Can you work these out from the model? Positions are in its coordinate system, mm. Face numbers are marked on the shaded views. A direction names the side the tool comes from. Give positions to 0.01 mm unless a question says otherwise; leave off trailing zeros. Loops run counter-clockwise (first coordinate to the right, second up) from the corner with the lowest first, then second, coordinate; pieces in that order, holes last. Notation, with made-up numbers: (41.25, 84.5) - (96.25, 84.5) arc R6 cw to (96.25, 91.5) - close; hole circle Ø9 at (27, -2.5). An arc over 180 degrees is marked (long way). Answer as a JSON object with one key per item and string values. Group by question number.
Item 1: Which directions (+Z, -Z, +X, -X, +Y, -Y) give clear straight access to the entire face, cutting with the end or side of a thin tool? Please do the marked faces 1, 2 and 3.
Item 2: Suppose I cut it at D-D on x = -12. Write out the boundary of the cut face in (y, z).
Item 3: Suppose I cut it at A-A on y = 0. Write out the boundary of the cut face in (x, z).
Item 4: Will these pins go through, and if not, where does the flat tip stop? pin 1 (20 mm diameter, centred on x = 0, y = 0, fed in from +Z); pin 2 (3 mm diameter, centred on y = 16.5, z = 3, fed in from +X); pin 3 (3 mm diameter, centred on y = 5, z = 2, fed in from -X); pin 4 (2 mm diameter, centred on y = 12, z = 2.5, fed in from -X).
Item 5: Suppose I cut it at B-B on x = -25. Write out the boundary of the cut face in (y, z).
Item 6: Please list where these lines run through material, in increasing order: L1, parallel to X at y = 14.5, z = 6; L2, parallel to X at y = -16.5, z = 3; L3, parallel to Y at x = -3.5, z = 3.
Item 7: Thinking about a two-plate mould opening in X: for the marked faces 4, 5 and 6, which applies, pulls with the +X half, pulls with the -X half, needs draft (parallel to the pull), parting line crosses it, or undercut?
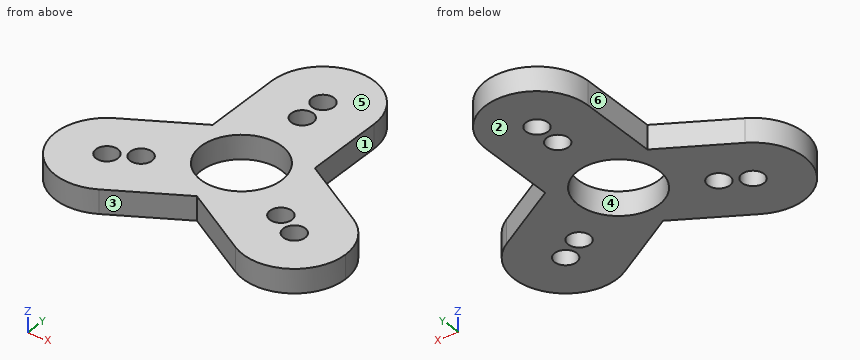
from build123d import *

# Parameters (mm, degrees)
F0_R     = 3
F0_R_2   = 11.05
F1_DEPTH = 6.5


with BuildPart() as f1:
    # F0 (on Top) → F1 (new body)
    with BuildSketch(Plane.XY):
        with BuildLine():
            ThreePointArc((-32.6519768305, -2.6858200754), (-37.7763321694, -21.8101758986), (-18.6519763031, -26.9345310768))
            ThreePointArc((-18.6519763031, -26.9345310768), (-13.5276209102, -21.8101754521), (-11.6519766687, -14.8101756349))
            ThreePointArc((-11.6519766687, -14.8101756349), (-18.6519767496, -2.6858199352), (-32.6519768305, -2.6858200754))
        make_face()
        with Locations((-25.6519766687, -14.8101756349)):
            Circle(F0_R, mode=Mode.SUBTRACT)
        with Locations((-19.1362317873, -11.0483085737)):
            Circle(F0_R, mode=Mode.SUBTRACT)
        with BuildLine():
            Line((0, -16.1658075373), (-7, -12.124355653))
            ThreePointArc((-7, -12.124355653), (-12.124355653, -7), (-14, 0))
            Line((-14, 0), (-14, 8.0829037687))
            Line((-14, 8.0829037687), (-32.6519768305, -2.6858200754))
            ThreePointArc((-32.6519768305, -2.6858200754), (-18.6519767496, -2.6858199352), (-11.6519766687, -14.8101756349))
            ThreePointArc((-11.6519766687, -14.8101756349), (-13.5276209102, -21.8101754521), (-18.6519763031, -26.9345310768))
            Line((-18.6519763031, -26.9345310768), (0, -16.1658075373))
        make_face()
        with BuildLine():
            Line((0, -16.1658075373), (7, -12.124355653))
            ThreePointArc((7, -12.124355653), (0, -14), (-7, -12.124355653))
            Line((-7, -12.124355653), (0, -16.1658075373))
        make_face()
        with BuildLine():
            ThreePointArc((39.6519766687, -14.8101756349), (37.7763323684, -7.8101757158), (32.6519768305, -2.6858200754))
            ThreePointArc((32.6519768305, -2.6858200754), (13.5276209927, -7.8101756747), (18.6519769101, -26.9345314273))
            ThreePointArc((18.6519769101, -26.9345314273), (32.6519767894, -26.9345312182), (39.6519766687, -14.8101756349))
        make_face()
        with Locations((19.1362317873, -11.0483085737)):
            Circle(F0_R, mode=Mode.SUBTRACT)
        with Locations((25.6519766687, -14.8101756349)):
            Circle(F0_R, mode=Mode.SUBTRACT)
        with BuildLine():
            Line((14, 8.0829037687), (14, 0))
            ThreePointArc((14, 0), (12.124355653, -7), (7, -12.124355653))
            Line((7, -12.124355653), (0, -16.1658075373))
            Line((0, -16.1658075373), (18.6519769101, -26.9345314273))
            ThreePointArc((18.6519769101, -26.9345314273), (13.5276209927, -7.8101756747), (32.6519768305, -2.6858200754))
            Line((32.6519768305, -2.6858200754), (14, 8.0829037687))
        make_face()
        with BuildLine():
            ThreePointArc((-14, 29.6203512698), (0, 15.6203512698), (14, 29.6203512698))
            ThreePointArc((14, 29.6203512698), (0, 43.6203512698), (-14, 29.6203512698))
        make_face()
        with Locations((0, 22.0966171473)):
            Circle(F0_R, mode=Mode.SUBTRACT)
        with Locations((0, 29.6203512698)):
            Circle(F0_R, mode=Mode.SUBTRACT)
        with BuildLine():
            ThreePointArc((-7, 12.124355653), (0, 14), (7, 12.124355653))
            Line((7, 12.124355653), (14, 8.0829037687))
            Line((14, 8.0829037687), (14, 29.6203512698))
            ThreePointArc((14, 29.6203512698), (0, 15.6203512698), (-14, 29.6203512698))
            Line((-14, 29.6203512698), (-14, 8.0829037687))
            Line((-14, 8.0829037687), (-7, 12.124355653))
        make_face()
        with BuildLine():
            ThreePointArc((-14, 0), (-12.124355653, 7), (-7, 12.124355653))
            Line((-7, 12.124355653), (-14, 8.0829037687))
            Line((-14, 8.0829037687), (-14, 0))
        make_face()
        with BuildLine():
            ThreePointArc((7, -12.124355653), (12.124355653, -7), (14, 0))
            ThreePointArc((14, 0), (12.124355653, 7), (7, 12.124355653))
            ThreePointArc((7, 12.124355653), (0, 14), (-7, 12.124355653))
            ThreePointArc((-7, 12.124355653), (-12.124355653, 7), (-14, 0))
            ThreePointArc((-14, 0), (-12.124355653, -7), (-7, -12.124355653))
            ThreePointArc((-7, -12.124355653), (0, -14), (7, -12.124355653))
        make_face()
        Circle(F0_R_2, mode=Mode.SUBTRACT)
        with BuildLine():
            ThreePointArc((7, 12.124355653), (12.124355653, 7), (14, 0))
            Line((14, 0), (14, 8.0829037687))
            Line((14, 8.0829037687), (7, 12.124355653))
        make_face()
    extrude(amount=F1_DEPTH)


solid = f1.part
Worked out:
{
 "1": {"face 1": "+Z, -Z, +X, +Y", "face 2": "-Z, +X, -X, +Y, -Y", "face 3": "+Z, -Z, -Y"},
 "2": {"outline": "(-23.09, 0) - (36.83, 0) - (36.83, 6.5) - (-23.09, 6.5) - close"},
 "3": {"outline": "(-28, 0) - (-11.05, 0) - (-11.05, 6.5) - (-28, 6.5) - close; (11.05, 0) - (28, 0) - (28, 6.5) - (11.05, 6.5) - close"},
 "4": {"pin 1": "passes through", "pin 2": "stops at x = 14", "pin 3": "stops at x = -21.94", "pin 4": "stops at x = -14"},
 "5": {"outline": "(-28.79, 0) - (-17.74, 0) - (-17.74, 6.5) - (-28.79, 6.5) - close; (-11.88, 0) - (1.73, 0) - (1.73, 6.5) - (-11.88, 6.5) - close"},
 "6": {"L1": "x = -14 to 14", "L2": "x = -39.55 to -28.13, -23.17 to -0.58, 0.58 to 23.17, 28.13 to 39.55", "L3": "y = -18.19 to -10.48, 10.48 to 43.18"},
 "7": {"face 4": "undercut", "face 5": "needs draft", "face 6": "pulls with the -X half"}
}
